The listing builds one solid part. Answer for the finished solid, in the listing's coordinates (mm). Face numbers are marked on the shaded views. A direction names the side the tool comes from. Coordinates: 2 decimals unless noted, no trailing zeros. Write each loop counter-clockwise with the first axis right and the second up, starting at its lowest first coordinate (ties: lowest second). Pieces come first, ordered by that corner, then holes.
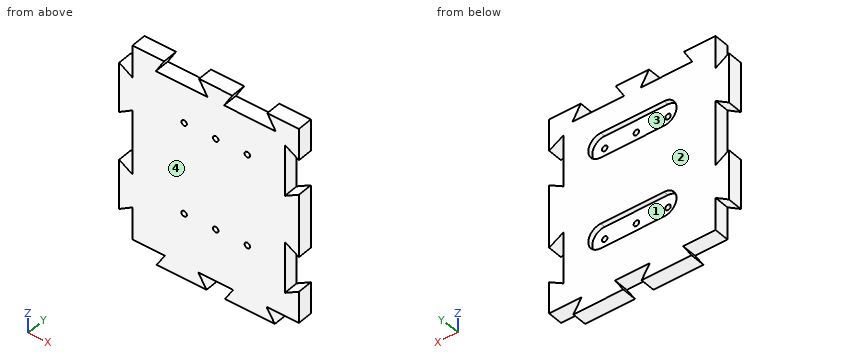
from build123d import *

# Parameters (mm, degrees)
SKETCH2_R           = 1.65
BOSS_EXTRUDE2_DEPTH = 9
CUT_EXTRUDE1_DEPTH  = 3


with BuildPart() as part:
    # Sketch2 → Boss-Extrude2 (new body)
    with BuildSketch(Plane(origin=(0, 0, 0), x_dir=(1, 0, 0), z_dir=(0, 1, 0))):
        Polygon((0, 98.5), (-8, 103.5), (-8, 73.5), (0, 78.5), (0, 39.5), (-8, 44.5), (-8, 14.5), (0, 19.5), (0, 0), (19, 0), (14, 8.5), (45, 8.5), (40, 0), (60, 0), (55, 8.5), (86, 8.5), (81, 0), (100, 0), (100, 19), (91.5, 14), (91.5, 45), (100, 40), (100, 78), (91.5, 73), (91.5, 104), (100, 99), (100, 118), (80.5, 118), (85.5, 126), (55.5, 126), (60.5, 118), (39.5, 118), (44.5, 126), (14.5, 126), (19.5, 118), (0, 118), align=None)
        with Locations(Location((31, 31.4, 0), (0, 0, 270))):
            Circle(SKETCH2_R, mode=Mode.SUBTRACT)
        with Locations(Location((31, 86.6, 0), (0, 0, 270))):
            Circle(SKETCH2_R, mode=Mode.SUBTRACT)
        with Locations(Location((50, 31.4, 0), (0, 0, 270))):
            Circle(SKETCH2_R, mode=Mode.SUBTRACT)
        with Locations(Location((50, 86.6, 0), (0, 0, 270))):
            Circle(SKETCH2_R, mode=Mode.SUBTRACT)
        with Locations(Location((69, 31.4, 0), (0, 0, 270))):
            Circle(SKETCH2_R, mode=Mode.SUBTRACT)
        with Locations(Location((69, 86.6, 0), (0, 0, 270))):
            Circle(SKETCH2_R, mode=Mode.SUBTRACT)
    extrude(amount=BOSS_EXTRUDE2_DEPTH)

    # Sketch4 → Cut-Extrude1 (cut)
    with BuildSketch(Plane(origin=(0, 9, 0), x_dir=(1, 0, 0), z_dir=(0, 1, 0))):
        with BuildLine():
            Line((31, 94.1), (69, 94.1))
            ThreePointArc((69, 94.1), (76.5, 86.6), (69, 79.1))
            Line((69, 79.1), (31, 79.1))
            ThreePointArc((31, 79.1), (23.5, 86.6), (31, 94.1))
        make_face()
        with BuildLine():
            Line((31, 38.9), (69, 38.9))
            ThreePointArc((69, 38.9), (76.5, 31.4), (69, 23.9))
            Line((69, 23.9), (31, 23.9))
            ThreePointArc((31, 23.9), (23.5, 31.4), (31, 38.9))
        make_face()
    extrude(amount=-CUT_EXTRUDE1_DEPTH, mode=Mode.SUBTRACT)


solid = part.part
Q1. The part is cut by section D-D, the plane y = 2.5. State how many separate pieces and enclosed holes the cut face has, then the cut area to 3 significant figures.
Answers below:
separate pieces: 1
enclosed holes: 6
area: 11,700 mm2
Q2. The part is cut by section C-C, the plane x = 50. Write down the section's boundary in (y, z), then the cut area to 3 significant figures.
Answers below:
outline: (0, -118) - (9, -118) - (9, -94.1) - (6, -94.1) - (6, -88.25) - (0, -88.25) - close; (0, -84.95) - (6, -84.95) - (6, -79.1) - (9, -79.1) - (9, -38.9) - (6, -38.9) - (6, -33.05) - (0, -33.05) - close; (0, -29.75) - (6, -29.75) - (6, -23.9) - (9, -23.9) - (9, 0) - (0, 0) - close
area: 932 mm2
Q3. Find the intervals of material crossed by probe 1 along Z at (x, y) = (69, 1.95); probe 2 along Z at (x, y) = (50, 4.35); probe 3 along X at (y, z) = (2.6, -31.4), in increasing order.
Answers below:
probe 1: z = -126 to -88.25, -84.95 to -33.05, -29.75 to -8.5
probe 2: z = -118 to -88.25, -84.95 to -33.05, -29.75 to 0
probe 3: x = -8 to 29.35, 32.65 to 48.35, 51.65 to 67.35, 70.65 to 91.5
Q4. Given pin 1 (7.5 mm diameter, centred on x = 55, z = -32.5, fed in from +Y); pin 2 (2.5 mm diameter, centred on y = 4.5, z = -91.5, fed in from +X); pin 3 (1 mm diameter, centred on y = 3, z = -62.5, fed in from -X), each flat-ended and moving along its own axis, determine where each tip first touches the part or whether it passes through.
Answers below:
pin 1: stops at y = 6
pin 2: stops at x = 91.5
pin 3: stops at x = 0
Q5. The part is cut by section B-B, the plane z = -86.6. Write down the section's boundary in (x, y).
Answers below:
outline: (-8, 0) - (29.35, 0) - (29.35, 6) - (23.5, 6) - (23.5, 9) - (-8, 9) - close; (32.65, 0) - (48.35, 0) - (48.35, 6) - (32.65, 6) - close; (51.65, 0) - (67.35, 0) - (67.35, 6) - (51.65, 6) - close; (70.65, 0) - (91.5, 0) - (91.5, 9) - (76.5, 9) - (76.5, 6) - (70.65, 6) - close
Q6. Determine the mould class of the marked faces 1 and 2 for opening direction X: released by +X, released by -X, zero draft, split by the parting line, or undercut.
Answers below:
face 1: undercut
face 2: zero draft
Q7. Which of the six approach directions +Z, -Z, +X, -X, +Y, -Y give full straight-line access (tool end or side, diameter ignored) to the marked faces 3 and 4?
Answers below:
face 3: +Y
face 4: +Z, -Z, +X, -X, -Y
Q8. The part is cut by section A-A, the plane z = -100.5. Write down the section's boundary in (x, y), then the cut area to 3 significant figures.
Answers below:
outline: (-8, 0) - (-3.2, 0) - (-3.2, 9) - (-8, 9) - close; (0, 0) - (91.5, 0) - (91.5, 9) - (0, 9) - close; (97.45, 0) - (100, 0) - (100, 9) - (97.45, 9) - close
area: 890 mm2
